Autodesk Inventor part; units mm, degrees
ref_plane "YZ Plane" through (0, 0, 0) normal (1, 0, 0) x (0, 1, 0)
ref_plane "XZ Plane" through (0, 0, 0) normal (0, 1, 0) x (-1, 0, 0)
ref_plane "XY Plane" through (0, 0, 0) normal (0, 0, 1) x (1, 0, 0)
sketch "Szkic1" plane through (0, 0, 0) normal (0, 1, 0) x (-1, 0, 0)
  line L0 (-60, -30) -> (60, -30)
  line L1 (60, -30) -> (60, 30)
  line L2 (60, 30) -> (-60, 30)
  line L3 (-60, 30) -> (-60, -30)
  line L4 (-60, -30) -> (60, 30) construction
  line L5 (60, -30) -> (-60, 30) construction
  point P0 (0, 0)
  dimension "d0" = 120
  dimension "d1" = 60
extrude "Płyta1" add sketch "Szkic1" along normal blind 2
sketch "Szkic2" plane through (60, 2, 30) normal (0, 0, 1) x (1, 0, 0)
  line L0 (-120, 0) -> (0, 0)
  line L1 (0, 0) -> (0, 41)
  line L2 (0, 41) -> (-120, 41)
  line L3 (-120, 41) -> (-120, 0)
edge flange "Kołnierz1" height 43 angle 90 thickness 2 bend radius 2.5 thickness toward (0, 0, 1) relief tear relief width 2 relief depth 1 corner gap 2 corner form 0 edges at (0, 2, 30) (0, 2, -30) wall of the first edge with corners at (-60, 2, 30) (60, 2, 30) (60, 43, 30) (-60, 43, 30)
bend "Zagięcie1"
corner "Narożnik1"
sketch "Szkic3" plane through (0, 2, 0) normal (0, 1, 0) x (1, 0, 0)
  circle A0 centre (48.5, 22) radius 1.2295
  circle A1 centre (48.5, -22) radius 1.2295
  circle A2 centre (-48.5, 22) radius 1.2295
  circle A3 centre (-48.5, -22) radius 1.2295
  point P0 (0, 0)
hole "Otwór1" at (48.5, 2, -22) at (48.5, 2, 22) at (-48.5, 2, -22) at (-48.5, 2, 22) direction (0, -1, 0) diameter 3.5 depth 2 tip angle 118
fillet "Zaokrąglenie1" radius 4 4 edges at (-60, 43, -31) (-60, 43, 31) (60, 43, 31) (60, 43, -31)
sketch "Szkic4" plane through (0, 0, 0) normal (0, -1, 0) x (1, 0, 0)
  circle A0 centre (-20, 0) radius 4
  circle A1 centre (-35, 17.5) radius 4
  circle A2 centre (-35, -17.5) radius 4
  line L0 (-60, -27.5) -> (-60, 27.5)
  point P0 (0, 0)
  dimension "d22" = 35
  dimension "d23" = 17.5
  dimension "d24" = 15
  dimension "d25" = 8
  dimension "d26" = 25
extrude "Wytnij1" cut sketch "Szkic4" against normal blind 2
sketch "Szkic5" plane through (0, 0, 0) normal (0, -1, 0) x (1, 0, 0)
  circle A0 centre (30, 0) radius 6
  line L0 (60, 27.5) -> (60, -27.5)
  point P0 (0, 0)
  point P1 (60, 0)
  dimension "d29" = 12
  dimension "d30" = 30
extrude "Wytnij2" cut sketch "Szkic5" against normal blind 2
sketch "Szkic6" plane through (60, 4.5, -32) normal (0, 0, -1) x (-1, 0, 0)
  circle A0 centre (50, 28.5) radius 5
  line L0 (4, 38.5) -> (116, 38.5)
  line L1 (0, 0) -> (0, 34.5)
  point P0 (60, -4.5)
  dimension "d33" = 10
  dimension "d34" = 10
  dimension "d35" = 50
extrude "Wytnij3" cut sketch "Szkic6" against normal through all
sketch "Szkic7" plane through (0, 0, 0) normal (0, -1, 0) x (1, 0, 0)
  circle A0 centre (-37, 0) radius 4
  line L0 (-60, -27.5) -> (-60, 27.5)
  point P0 (0, 0)
  point P1 (-60, 0)
  dimension "d38" = 8
  dimension "d39" = 23
extrude "Wytnij4" cut sketch "Szkic7" against normal blind 2
sketch "Szkic8" plane through (-60, 4.5, 32) normal (0, 0, 1) x (1, 0, 0)
  circle A0 centre (95, 23.5) radius 6
  line L0 (120, 34.5) -> (120, 0)
  circle A1 centre (70, 28.5) radius 5
  line L1 (4, 38.5) -> (116, 38.5)
  point P0 (60, -4.5)
  dimension "d42" = 12
  dimension "d43" = 25
  dimension "d46" = 15
extrude "Wytnij5" cut sketch "Szkic8" against normal blind 2 contours A0
equation "\"d19\" = Grubość"
equation "\"d27\" = Grubość"
equation "\"d31\" = Grubość"
equation "\"d36\" = Grubość"
equation "\"d40\" = Grubość"
equation "\"d44\" = Grubość"
equation "\"d2\" = Grubość"
equation "\"d3\" = SzerokośćGięciaPodcięcia"
equation "\"d4\" = GłębokośćGięciaPodcięcia"
equation "\"d5\" = MinimalnaPozostałość"
equation "\"d6\" = PromieńPrzejścia"
equation "\"d10\" = RozmiarPodcięciaNarożnika"
equation "\"d11\" = Wielk_odstępu"
equation "\"d12\" = Rozmiar_promienia_Jacobiego"
equation "\"PromieńGięcia\" = Grubość"
equation "\"SzerokośćGięciaPodcięcia\" = Grubość"
equation "\"GłębokośćGięciaPodcięcia\" = 0.5 * Grubość"
equation "\"RozmiarPodcięciaNarożnika\" = 4 * Grubość"
equation "\"MinimalnaPozostałość\" = 2 * Grubość"
equation "\"PromieńPrzejścia\" = PromieńGięcia"
equation "\"Rozmiar_promienia_Jacobiego\" = PromieńGięcia"
equation "\"Wielk_odstępu\" = Grubość"
properties part number "dekiel" material "Stal"
Source: CAD feature listing. Evaluate the final solid. Frame: model axes, mm. A direction names the side the tool comes from. Give positions to 0.01 mm unless a question says otherwise; leave off trailing zeros. Write each loop counter-clockwise with the first axis right and the second up, starting at its lowest first coordinate (ties: lowest second). Pieces come first, ordered by that corner, then holes. Notation, with made-up numbers: (-25.5, 83.25) - (23.5, 83.25) arc R28 cw to (23.5, 119.25) - close; hole circle Ø11 at (69, -12). An arc over 180 degrees is marked (long way). One line per item, written item: value. Start each with the question number.
Q1. First-contact query: pin 1 Ø6.5 at (x, z) = (-35, -17.5) entering from +Y; pin 2 Ø5.5 at (x, z) = (48.5, 22) entering from +Y; pin 3 Ø11 at (x, y) = (35, 28) entering from +Z. Flat tips, straight axial feed; report the tip coordinate or a pass-through.
Q2. Section query C-C, the plane y = 20. Return the cut outline in (x, z), then the cut area to 3 significant figures.
Q3. Section query D-D, the plane y = 29.5. Return the cut outline in (x, z).
Q4. Section query B-B, the plane z = 17.5. Return the cut outline in (x, y), then the cut area to 3 significant figures.
Q5. Section query A-A, the plane x = -48.5. Return the cut outline in (y, z).
Q6. Material intervals for probe 1 along Z at (x, y) = (-34, 33); probe 2 along X at (y, z) = (1, -22); probe 3 along Z at (x, y) = (-48.5, 0.6) (3 decimals), sorted ascending. Write a range as from..to.
Q7. Set-up query: faces 1 (the face through (-58.797, 41.859, 31.014)), 2 (the face through (-0.84, 2.752, -29.287)). Return all of +Z, -Z, +X, -X, +Y, -Y with unobstructed straight access to the full face (end or side cutting, diameter ignored); none if empty.
Q8. Draft query along Y for faces 3 (the face through (5.23, 34.5, -31.01)), 4 (the face through (1, 0, 0)), 5 (the face through (-23.2, 1, -2.4)), 6 (the face through (30.24, 24.35, 31.01)). Return one class per face: +Y half, -Y half, draft (parallel to the pull), parting line (faces both ways), or undercut.
Answer:
1. pin 1: passes through
1. pin 2: stops at y = 2
1. pin 3: stops at z = -30
2. outline: (-60, -32) - (60, -32) - (60, -30) - (-60, -30) - close; (-60, 30) - (60, 30) - (60, 32) - (-60, 32) - close
2. area: 480 mm2
3. outline: (-60, -32) - (6.43, -32) - (6.43, -30) - (-60, -30) - close; (-60, 30) - (6.43, 30) - (6.43, 32) - (-60, 32) - close; (13.57, -32) - (60, -32) - (60, -30) - (13.57, -30) - close; (13.57, 30) - (29.19, 30) - (29.19, 32) - (13.57, 32) - close; (40.81, 30) - (60, 30) - (60, 32) - (40.81, 32) - close
4. outline: (-60, 0) - (-39, 0) - (-39, 2) - (-60, 2) - close; (-31, 0) - (60, 0) - (60, 2) - (-31, 2) - close
4. area: 224 mm2
5. outline: (0, -27.5) arc R4.5 ccw to (4.5, -32) - (43, -32) - (43, -30) - (4.5, -30) arc R2.5 cw to (2, -27.5) - (2, -23.75) - (0, -23.75) - close; (0, -20.25) - (2, -20.25) - (2, 20.25) - (0, 20.25) - close; (0, 23.75) - (2, 23.75) - (2, 27.5) arc R2.5 cw to (4.5, 30) - (43, 30) - (43, 32) - (4.5, 32) arc R4.5 ccw to (0, 27.5) - close
6. probe 1: z = -32..-30, 30..32
6. probe 2: x = -60..-50.25, -46.75..46.75, 50.25..60
6. probe 3: z = -29.745..-23.75, -20.25..20.25, 23.75..29.745
7. face 1: +Z, -Z, -X, +Y
7. face 2: +X, -X, +Y
8. face 3: undercut
8. face 4: -Y half
8. face 5: draft
8. face 6: undercut
